from build123d import *

# Parameters (mm, degrees)
EXTRUDE_1_DEPTH     = 8
SKETCH_2_W          = 4
SKETCH_2_H          = 2
CUT_EXTRUDE_1_DEPTH = 14.304134696
SKETCH_3_W          = 4
SKETCH_3_H          = 2
CUT_EXTRUDE_2_DEPTH = 14.304134696
SKETCH_4_W          = 3
SKETCH_4_H          = 14
CHAMFER_1_SIZE      = 0.500002905
CHAMFER_1_SIZE2     = 0.500003995
FILLET_1_R          = 1
FILLET_2_R          = 2
FILLET_3_R          = 3
FILLET_4_R          = 4


with BuildPart() as part:
    # 草图1 → 凸台-拉伸1 (new body)
    with BuildSketch(Plane(origin=(0, 4, 0), x_dir=(1, 0, 0), z_dir=(0, 1, 0))):
        Polygon((-8, -7), (8, -7), (8, -2.5), (5.5, 0), (-5.5, 0), (-8, -2.5), align=None)
    extrude(amount=-EXTRUDE_1_DEPTH)

    # 草图2 → 切除-拉伸1 (cut, through all)
    with BuildSketch(Plane.XZ.offset(4)):
        with Locations((-6, 6)):
            Rectangle(SKETCH_2_W, SKETCH_2_H)
    extrude(amount=-CUT_EXTRUDE_1_DEPTH, mode=Mode.SUBTRACT)

    # 草图3 → 切除-拉伸2 (cut, through all)
    with BuildSketch(Plane.XZ.offset(4)):
        with Locations((6, 6)):
            Rectangle(SKETCH_3_W, SKETCH_3_H)
    extrude(amount=-CUT_EXTRUDE_2_DEPTH, mode=Mode.SUBTRACT)

    # 草图4 → 旋转1 (revolve)
    with BuildSketch(Plane(origin=(0, 0, 0), x_dir=(1, 0, 0), z_dir=(0, 1, 0))):
        with Locations((1.5, -14)):
            Rectangle(SKETCH_4_W, SKETCH_4_H)
    revolve(axis=Axis((0, 0, 7), (0, 0, 1)))

    # 倒角1
    chamfer_1_edges = [part.edges().sort_by_distance(p)[0] for p in [
        (-3, 0, 21),
    ]]
    chamfer_1_side = [part.faces().sort_by_distance(p)[0] for p in [
        (-3, 0, 14),
    ]]
    chamfer(chamfer_1_edges, length=CHAMFER_1_SIZE, length2=CHAMFER_1_SIZE2, reference=chamfer_1_side[0])

    # 圆角1
    fillet_1_edges = [part.edges().sort_by_distance(p)[0] for p in [
        (8, 4, 3.75),
        (-8, -4, 3.75),
    ]]
    fillet(fillet_1_edges, radius=FILLET_1_R)

    # 圆角2
    fillet_2_edges = [part.edges().sort_by_distance(p)[0] for p in [
        (-5.5, 0, 0),
        (5.5, 0, 0),
    ]]
    fillet(fillet_2_edges, radius=FILLET_2_R)

    # 圆角3
    fillet_3_edges = [part.edges().sort_by_distance(p)[0] for p in [
        (8, -4, 3.75),
        (-8, 4, 3.75),
    ]]
    fillet(fillet_3_edges, radius=FILLET_3_R)

    # 圆角4
    fillet_4_edges = [part.edges().sort_by_distance(p)[0] for p in [
        (-4, 4, 6),
        (4, -4, 6),
    ]]
    fillet(fillet_4_edges, radius=FILLET_4_R)


solid = part.part
For this review, take the finished solid that the model builds, in its own axes (mm). A direction names the side the tool comes from. Round coordinates to 2 decimals unless told otherwise and drop trailing zeros. Write each loop counter-clockwise with the first axis right and the second up, starting at its lowest first coordinate (ties: lowest second). Pieces come first, ordered by that corner, then holes. Notation, with made-up numbers: (80.25, 44.25) -> (113.25, 44.25) arc R28 cw to (113.25, 77.25) -> close; hole circle Ø3 at (51.5, 35.25). An arc over 180 degrees is marked (long way). Use CSV: the item, a comma, the result in double quotes.
(1) Clearance check with flat-ended pins moving along their axes: P1, Ø1.5, axis at x = -1.5, z = 16.5, coming from the -Y side; P2, Ø1, axis at y = 3, z = 11, coming from the +X side; P3, Ø1, axis at y = -2.5, z = 6.5, coming from the -X side. State where each tip first meets the part, or that it passes through.
Computed values:
P1,"y = -2.9"
P2,"x = 1.66"
P3,"x = -4"
(2) To check wall thickness, follow L1, parallel to Z at x = -5, y = -1.5; L2, parallel to Z at x = 3.5, y = 2.5; L3, parallel to X at y = -1.5, z = 5.5. State the ranges of each line that lie inside material, in increasing order. Write a range as [from, to].
Computed values:
L1,"[0.03, 5]"
L2,"[0, 7]"
L3,"[-4, 3.71]"
(3) For faces 1 (the face through (4, 2, 6)), 2 (the face through (3, -2, 7)), 3 (the face through (-4, -2, 6)), list the 3-axis set-ups (+Z, -Z, +X, -X, +Y, -Y) from which the entire face can be reached by the end or side of a thin tool; tool diameter is ignored.
Computed values:
face 1,"+Z, +X, +Y, -Y"
face 2,"+Z"
face 3,"+Z, -X, +Y, -Y"
(4) Consider section A-A, the plane z = 14.75. Give the boundary of the cut face in (x, y).
Computed values:
outline,"circle Ø6 at (0, 0)"
(5) Consider section B-B, the plane x = -5.25. Give the boundary of the cut face in (y, z).
Computed values:
outline,"(-4, 0.09) -> (3.99, 0.09) -> (3.99, 5) -> (-4, 5) -> close"
